For this review, take the finished solid that the model builds, in its own axes (mm). Give positions to 0.01 mm unless a question says otherwise; leave off trailing zeros. Order: outer loops, then holes, each group sorted by start corner. A loop starts at its lowest first (then second) coordinate and runs counter-clockwise, first axis right, second up.
from build123d import *

# Parameters (mm, degrees)
SKETCH_1_W      = 12
SKETCH_1_H      = 6
SKETCH_1_W_2    = 6
EXTRUDE_1_DEPTH = 6


with BuildPart() as part:
    # Эскиз1 → Бобышка-Вытянуть1 (new body)
    with BuildSketch(Plane.XY):
        Polygon((100, 40), (150, 40), (150, 43), (200, 43), (200, 40), (250, 40), (250, 43), (300, 43), (300, 40), (350, 40), (350, 43), (400, 43), (400, 40), (450, 40), (450, 27.5), (444, 27.5), (444, 12.5), (450, 12.5), (450, 0), (0, 0), (0, 12.5), (6, 12.5), (6, 27.5), (0, 27.5), (0, 40), (50, 40), (50, 43), (100, 43), align=None)
        with Locations((19, 31)):
            Rectangle(SKETCH_1_W, SKETCH_1_H, mode=Mode.SUBTRACT)
        with Locations((431, 31)):
            Rectangle(SKETCH_1_W, SKETCH_1_H, mode=Mode.SUBTRACT)
        with Locations((248, 27)):
            Rectangle(SKETCH_1_W_2, SKETCH_1_H, mode=Mode.SUBTRACT)
        with Locations((248, 13)):
            Rectangle(SKETCH_1_W_2, SKETCH_1_H, mode=Mode.SUBTRACT)
        with Locations((202, 27)):
            Rectangle(SKETCH_1_W_2, SKETCH_1_H, mode=Mode.SUBTRACT)
        with Locations((202, 13)):
            Rectangle(SKETCH_1_W_2, SKETCH_1_H, mode=Mode.SUBTRACT)
    extrude(amount=EXTRUDE_1_DEPTH)


solid = part.part
1) Clearance check with flat-ended pins moving along their axes: pin 1 (1.5 mm diameter, centred on y = 41.5, z = 2, fed in from -X); pin 2 (3 mm diameter, centred on x = 202.5, z = 4, fed in from +Y). State where each tip first meets the part, or that it passes through.
Answer sheet:
pin 1: stops at x = 50
pin 2: stops at y = 40
2) We need section B-B on z = 4.95. Count the separate pieces of the cut face and the enclosed holes in it, then the cut area to 3 significant figures.
Answer sheet:
separate pieces: 1
enclosed holes: 6
area: 18,100 mm2
3) We need section A-A on x = 43. Give the boundary of the cut face in (y, z), then the cut area to 3 significant figures.
Answer sheet:
outline: (0, 0) - (40, 0) - (40, 6) - (0, 6) - close
area: 240 mm2
4) To check wall thickness, follow line 1 (X direction, y = 12, z = 1.7); line 2 (X direction, y = 25, z = 5); line 3 (Y direction, x = 18, z = 1.6). State the ranges of each line that lie inside material, in increasing order.
Answer sheet:
line 1: x = 0 to 199, 205 to 245, 251 to 450
line 2: x = 6 to 199, 205 to 245, 251 to 444
line 3: y = 0 to 28, 34 to 40
